Autodesk Fusion 360 part; units mm, degrees
sketch "Skizze1" plane through (0, 0, 0) normal (0, 0, 1) x (1, 0, 0)
  line L0 (8, 0) -> (92, 0)
  line L1 (100, 8) -> (100, 92)
  line L2 (92, 100) -> (8, 100)
  line L3 (0, 92) -> (0, 8)
  arc A0 (8, 100) -> (0, 92) centre (8, 92) ccw
  arc A1 (100, 92) -> (92, 100) centre (92, 92) ccw
  arc A2 (92, 0) -> (100, 8) centre (92, 8) ccw
  arc A3 (0, 8) -> (8, 0) centre (8, 8) ccw
  circle A4 centre (8, 8) radius 2
  circle A5 centre (92, 8) radius 2
  circle A6 centre (92, 92) radius 2
  circle A7 centre (8, 92) radius 2
  line L4 (70, 50) -> (70, 70)
  line L5 (70, 70) -> (50, 70)
  line L6 (70, 70) -> (30, 70)
  line L7 (30, 70) -> (30, 30)
  line L8 (30, 30) -> (70, 30)
  line L9 (70, 30) -> (70, 70)
  line L10 (0, 100) -> (9.4142, 90.5858)
  line L11 (90.5858, 9.4142) -> (100, 0)
  circle A8 centre (25, 75) radius 1.9
  circle A9 centre (75, 75) radius 1.9
  circle A10 centre (75, 25) radius 1.9
  circle A11 centre (25, 25) radius 1.9
  line L12 (80, 50) -> (80, 80)
  line L13 (80, 80) -> (50, 80)
  line L14 (80, 80) -> (20, 80)
  line L15 (20, 80) -> (20, 20)
  line L16 (20, 20) -> (80, 20)
  line L17 (80, 20) -> (80, 80)
  line L18 (17, 83) -> (83, 83)
  line L19 (83, 83) -> (83, 17)
  line L20 (83, 17) -> (17, 17)
  line L21 (17, 17) -> (17, 83)
  point P0 (100, 0)
  point P1 (0, 100)
  dimension "d1" = 100
  dimension "d2" = 100
  dimension "d3" = 8
  dimension "d4" = 4
  dimension "d5" = 4
  dimension "d6" = 4
  dimension "d9" = 40
  dimension "d10" = 40
  dimension "d11" = 3.8
  dimension "d12" = 3.8
  dimension "d13" = 3.8
  dimension "d14" = 3.8
extrude "Extrusion1" add sketch "Skizze1" along normal blind 2 contours L0 L1 L2 L3 A0 A1 A2 A3
extrude "Extrusion2" add sketch "Skizze1" along normal blind 5 contours L18 L19 L20 L21
extrude "Extrusion3" add sketch "Skizze1" along normal blind 2 contours L12 L13 L14 L15 L16 L17
extrude "Extrusion4" add sketch "Skizze1" along normal blind 19 contours A8 | A9 | A10 | A11
fillet "Abrundung1" radius 2.5 4 edges at (50, 17, 5) (17, 50, 5) (50, 83, 5) (83, 50, 5)
Design review of the part built by this model. Coordinates are the model's own, in mm. A direction names the side the tool comes from. Give positions to 0.01 mm unless a question says otherwise; leave off trailing zeros. Order: outer loops, then holes, each group sorted by start corner. A loop starts at its lowest first (then second) coordinate and runs counter-clockwise, first axis right, second up. Notation, with made-up numbers: (9.25, 35) - (63.25, 35) arc R26 ccw to (63.25, 74) - close; hole circle Ø5 at (-8, 51.25). An arc over 180 degrees is marked (long way). Use a Markdown table: item, result. Add a question column.
(1) Add section A-A on x = 51. Give the boundary of the cut face in (y, z), then the cut area to 3 significant figures.
(2) Wall thickness on probe 1 along Y at (x, z) = (92, 0.65); probe 2 along Y at (x, z) = (54.5, 1); probe 3 along Z at (x, y) = (70, 93): over which ranges is each line inside the solid? List them lowest first. Write a range as [from, to].
(3) Machinability: for faces 4 (the face through (24.588, 76.855, 10.381)), 5 (the face through (97.719, 2.406, 0.986)), which of the approach directions +Z, -Z, +X, -X, +Y, -Y give a long, thin tool a straight path to every point of the face, cutting with its end or side? Answer none if there is none.
(4) Mouldability with a two-part tool opening along X and no side actions: class faces 1 (the face through (2.406, 2.281, 0.986)), 2 (the face through (82.287, 49.538, 4.248)), 3 (the face through (8, 90, 1)) as +X half, -X half, draft (parallel to the pull), parting line (faces both ways), or undercut.
(5) Clearance check with flat-ended pins moving along their axes: P1, Ø2.5, axis at x = 56, z = 3.5, coming from the +Y side; P2, Ø3.5, axis at x = 92, y = 8, coming from the -Z side; P3, Ø1, axis at x = 13.5, y = 46.5, coming from the +Z side; P4, Ø5, axis at x = 59, y = 83, coming from the +Z side. State where each tip first meets the part, or that it passes through.
(6) Add section C-C on y = 25. Give the boundary of the cut face in (x, z), then the cut area to 3 significant figures.
(7) Add section D-D on z = 7. Give the boundary of the cut face in (x, y), then the cut area to 3 significant figures.
Report:
| question | item | result |
|---|---|---|
| 1 | outline | (0, 0) - (30, 0) - (30, 2) - (20, 2) - (20, 5) - (19.5, 5) arc R2.5 ccw to (17, 2.5) - (17, 2) - (0, 2) - close; (70, 0) - (100, 0) - (100, 2) - (83, 2) - (83, 2.5) arc R2.5 ccw to (80.5, 5) - (80, 5) - (80, 2) - (70, 2) - close |
| 1 | area | 135 mm² |
| 2 | probe 1 | y = [0, 6], [10, 90], [94, 100] |
| 2 | probe 2 | y = [0, 30], [70, 100] |
| 2 | probe 3 | z = [0, 2] |
| 3 | face 4 | +Z |
| 3 | face 5 | +Z, -Z, +X, -Y |
| 4 | face 1 | -X half |
| 4 | face 2 | +X half |
| 4 | face 3 | undercut |
| 5 | P1 | stops at y = 83 |
| 5 | P2 | passes through |
| 5 | P3 | stops at z = 2 |
| 5 | P4 | stops at z = 5 |
| 6 | outline | (0, 0) - (100, 0) - (100, 2) - (83, 2) - (83, 2.5) arc R2.5 ccw to (80.5, 5) - (80, 5) - (80, 2) - (76.9, 2) - (76.9, 19) - (73.1, 19) - (73.1, 2) - (26.9, 2) - (26.9, 19) - (23.1, 19) - (23.1, 2) - (20, 2) - (20, 5) - (19.5, 5) arc R2.5 ccw to (17, 2.5) - (17, 2) - (0, 2) - close |
| 6 | area | 345 mm² |
| 7 | outline | circle Ø3.8 at (25, 25); circle Ø3.8 at (25, 75); circle Ø3.8 at (75, 25); circle Ø3.8 at (75, 75) |
| 7 | area | 45.4 mm² |
